from build123d import *

# Parameters (mm, degrees)
SKETCH006_W          = 87.85
SKETCH006_H          = 45.25
PAD_DEPTH            = 2
SKETCH007_W          = 74.25
SKETCH007_H          = 2
PAD001_DEPTH         = 5
SKETCH008_W          = 87.85
SKETCH008_H          = 45.25
SKETCH008_W_2        = 2.6
SKETCH008_H_2        = 7.75
PAD002_DEPTH         = 25
SKETCH009_W          = 4.6
SKETCH009_H          = 2
PAD003_DEPTH         = 6
SKETCH010_W          = 3.4
SKETCH010_H          = 2
PAD004_DEPTH         = 18
SKETCH011_W          = 3.4
SKETCH011_H          = 2
PAD005_DEPTH         = 1.5
SKETCH013_W          = 4.6
SKETCH013_H          = 9.75
POCKET001_DEPTH      = 1
SKETCH016_R          = 2
POCKET003_DEPTH      = 2
POCKET003_DEPTH_BACK = 5
POCKET004_DEPTH      = 2
SKETCH044_R          = 1.75
PAD031_DEPTH         = 2
SKETCH070_R          = 1.95
POCKET_DEPTH         = 2
SKETCH086_R          = 1.5
POCKET019_DEPTH      = 2


with BuildPart() as part:
    # Sketch006 → Pad (new body)
    with BuildSketch(Plane.XY):
        with Locations((2.3, 0)):
            Rectangle(SKETCH006_W, SKETCH006_H)
    extrude(amount=PAD_DEPTH)

    # Sketch007 (on Face6 of Pad) → Pad001 (join)
    with BuildSketch(Plane.XY.offset(2)):
        with Locations((0, 17.125)):
            Rectangle(SKETCH007_W, SKETCH007_H)
        with Locations((0, -17.125)):
            Rectangle(SKETCH007_W, SKETCH007_H)
    extrude(amount=PAD001_DEPTH)

    # Sketch008 (on Face5 of Pad001) → Pad002 (join)
    with BuildSketch(Plane.XY.offset(2)):
        with Locations((2.3, 0)):
            Rectangle(SKETCH008_W, SKETCH008_H)
        Polygon((-39.625, 20.625), (39.625, 20.625), (39.625, 10.875), (44.225, 10.875), (44.225, -20.625), (-39.625, -20.625), align=None, mode=Mode.SUBTRACT)
        with Locations((42.925, 16.75)):
            Rectangle(SKETCH008_W_2, SKETCH008_H_2, mode=Mode.SUBTRACT)
    extrude(amount=PAD002_DEPTH)

    # Sketch009 (on Face6 of Pad) → Pad003 (join)
    with BuildSketch(Plane.XY.offset(2)):
        with Locations((41.925, 2.375)):
            Rectangle(SKETCH009_W, SKETCH009_H)
        with Locations((41.925, -12.625)):
            Rectangle(SKETCH009_W, SKETCH009_H)
    extrude(amount=PAD003_DEPTH)

    # Sketch010 (on Face26 of Pad003) → Pad004 (join)
    with BuildSketch(Plane.XY.offset(8)):
        with Locations((42.525, -12.625)):
            Rectangle(SKETCH010_W, SKETCH010_H)
    extrude(amount=PAD004_DEPTH)

    # Sketch011 (on Face23 of Pad003) → Pad005 (join)
    with BuildSketch(Plane.XY.offset(8)):
        with Locations((42.525, 2.375)):
            Rectangle(SKETCH011_W, SKETCH011_H)
    extrude(amount=PAD005_DEPTH)

    # Sketch013 (on Face9 of Pad002) → Pocket001 (cut)
    with BuildSketch(Plane.XY.offset(27)):
        with Locations((41.925, 15.75)):
            Rectangle(SKETCH013_W, SKETCH013_H)
    extrude(amount=-POCKET001_DEPTH, mode=Mode.SUBTRACT)

    # Sketch016 → Pocket003 (cut, two sides)
    with BuildSketch(Plane(origin=(-40.625, 0, 0), x_dir=(0, -1, 0), z_dir=(-1, 0, 0))) as pocket003_sk:
        with Locations((0, 6.5)):
            Circle(SKETCH016_R)
    extrude(amount=-POCKET003_DEPTH, mode=Mode.SUBTRACT)
    extrude(pocket003_sk.sketch, amount=POCKET003_DEPTH_BACK, mode=Mode.SUBTRACT)

    # Sketch017 (on Face5 of Pocket003) → Pocket004 (cut)
    with BuildSketch(Plane.XZ.offset(22.625)):
        with BuildLine():
            Line((40.325, 14), (40.325, 29))
            Line((40.325, 29), (43.825, 29))
            Line((43.825, 14), (43.825, 29))
            ThreePointArc((42.825, 13), (43.532107, 13.292893), (43.825, 14))
            Line((41.325, 13), (42.825, 13))
            ThreePointArc((40.325, 14), (40.617893, 13.292893), (41.325, 13))
        make_face()
    extrude(amount=-POCKET004_DEPTH, mode=Mode.SUBTRACT)

    # Sketch044 (on Face9 of Pad002) → Pad031 (join)
    with BuildSketch(Plane.XY.offset(27)):
        with BuildLine():
            ThreePointArc((-47.453427, 2.828427), (-48.625, 0), (-47.453427, -2.828427))
            Line((-47.453427, -2.828427), (-41.625, -8.656854))
            Line((-41.625, 8.656854), (-41.625, -8.656854))
            Line((-47.453427, 2.828427), (-41.625, 8.656854))
        make_face()
        with Locations((-44.625, 0)):
            Circle(SKETCH044_R, mode=Mode.SUBTRACT)
        with BuildLine():
            ThreePointArc((52.053427, -2.828427), (53.225, 0), (52.053427, 2.828427))
            Line((52.053427, 2.828427), (46.225, 8.656854))
            Line((46.225, -8.656854), (46.225, 8.656854))
            Line((52.053427, -2.828427), (46.225, -8.656854))
        make_face()
        with Locations((49.225, 0)):
            Circle(SKETCH044_R, mode=Mode.SUBTRACT)
    extrude(amount=-PAD031_DEPTH)

    # Sketch070 (on Face4 of Pad031) → Pocket (cut)
    with BuildSketch(Plane(origin=(0, 0, 0), x_dir=(1, 0, 0), z_dir=(0, 0, -1))):
        with Locations((-17.225, 0)):
            Circle(SKETCH070_R)
        with Locations((21.825, 0)):
            Circle(SKETCH070_R)
    extrude(amount=-POCKET_DEPTH, mode=Mode.SUBTRACT)

    # Sketch086 (on Face14 of Pad002) → Pocket019 (cut)
    with BuildSketch(Plane(origin=(44.225, 0, 0), x_dir=(0, -1, 0), z_dir=(-1, 0, 0))):
        with Locations((10.125, 12)):
            Circle(SKETCH086_R)
    extrude(amount=-POCKET019_DEPTH, mode=Mode.SUBTRACT)


with BuildPart() as part_1:
    # Body placement: moved
    add(part.part.moved(Location((0, 0, -2))))


solid = part_1.part
For this review, take the finished solid that the model builds, in its own axes (mm). A direction names the side the tool comes from. Coordinates: 2 decimals unless noted, no trailing zeros. Loops run counter-clockwise (first coordinate to the right, second up) from the corner with the lowest first, then second, coordinate; pieces in that order, holes last. Notation, with made-up numbers: (60.25, 76.5) -> (115.25, 76.5) arc R28 ccw to (115.25, 112.5) -> close; hole circle Ø4 at (46, 5.5). An arc over 180 degrees is marked (long way). Write each question's results on one line, items separated by ' | '.
Q1. Mouldability with a two-part tool opening along X and no side actions: class faces 1 (the flat face through (-44.58, -5.7, 24.01)), 2 (the flat face through (39.625, 2, 3)), 3 (the flat face through (2, 22, 25)), 4 (the flat face through (43, 17, 0)) as +X half, -X half, draft (parallel to the pull), parting line (faces both ways), or undercut.
Taken from the geometry:
face 1: -X half | face 2: undercut | face 3: draft | face 4: undercut
Q2. Add section A-A, the plane y = 0. Count the separate pieces of the cut face and the enclosed holes in it, then the cut area to 3 significant figures.
Taken from the geometry:
separate pieces: 6 | enclosed holes: 0 | area: 266 mm²
Q3. Add section B-B, the plane z = 21.75. State the section outline as (x, y) points (3 decimals).
Taken from the geometry:
outline: (-41.625, -22.625) -> (40.325, -22.625) -> (40.325, -20.625) -> (-39.625, -20.625) -> (-39.625, 20.625) -> (39.625, 20.625) -> (39.625, 10.875) -> (44.225, 10.875) -> (44.225, -11.625) -> (40.825, -11.625) -> (40.825, -13.625) -> (44.225, -13.625) -> (44.225, -20.625) -> (43.825, -20.625) -> (43.825, -22.625) -> (46.225, -22.625) -> (46.225, 22.625) -> (-41.625, 22.625) -> close; hole (41.625, 12.875) -> (44.225, 12.875) -> (44.225, 20.625) -> (41.625, 20.625) -> close
Q4. To check wall thickness, follow line 1 along X through (y, z) = (18, 16.25) (3 decimals); line 2 along X through (y, z) = (8.5, 11.25) (3 decimals); line 3 along Y through (x, z) = (-13, 6.25) (3 decimals). State the ranges of each line that lie inside material, in increasing order. Write a range as [from, to].
Taken from the geometry:
line 1: [-41.625, -39.625], [39.625, 41.625], [44.225, 46.225] | line 2: [-41.625, -39.625], [44.225, 46.225] | line 3: [-22.625, -20.625], [20.625, 22.625]
Q5. Add section D-D, the plane y = -5. State the section outline as (x, z) points (3 decimals), then the cut area to 3 significant figures.
Taken from the geometry:
outline: (-45.282, 23) -> (-41.625, 23) -> (-41.625, -2) -> (46.225, -2) -> (46.225, 23) -> (49.882, 23) -> (49.882, 25) -> (44.225, 25) -> (44.225, 0) -> (-39.625, 0) -> (-39.625, 25) -> (-45.282, 25) -> close | area: 290 mm²
Q6. Add section C-C, the plane x = -0.5. State the section outline as (y, z) points (3 decimals).
Taken from the geometry:
outline: (-22.625, -2) -> (22.625, -2) -> (22.625, 25) -> (20.625, 25) -> (20.625, 0) -> (18.125, 0) -> (18.125, 5) -> (16.125, 5) -> (16.125, 0) -> (-16.125, 0) -> (-16.125, 5) -> (-18.125, 5) -> (-18.125, 0) -> (-20.625, 0) -> (-20.625, 25) -> (-22.625, 25) -> close
Q7. For pin 1 Ø1 at (y, z) = (-15.5, 4) entering from -X (3 decimals); pin 2 Ø2 at (x, y) = (-44.625, 0) entering from -Z; pin 3 Ø5 at (y, z) = (-10.125, 10) entering from +X (3 decimals); pin 4 Ø12.5 at (x, y) = (-2.5, -10) entering from +Z, all flat-tipped, find the tip position at first contact; note any pin that passes through.
Taken from the geometry:
pin 1: x = -41.625 | pin 2: through | pin 3: x = 46.225 | pin 4: z = 5
Q8. Machinability: for faces 5 (the cylindrical face through (50.84, -0.67, 24.01)), 6 (the flat face through (37.125, 17, 2)), 7 (the cylindrical face through (45.211, -8.935, 9.087)), 8 (the flat face through (-44, -2, 23)), which of the approach directions +Z, -Z, +X, -X, +Y, -Y give a long, thin tool a straight path to every point of the face, cutting with its end or side? Answer none if there is none.
Taken from the geometry:
face 5: +Z, -Z | face 6: +Z | face 7: +X | face 8: -Z, -X, +Y, -Y
